The model under review builds one solid part; all positions refer to its coordinate system, in mm. A direction names the side the tool comes from. Coordinates: 2 decimals unless noted, no trailing zeros. Loops run counter-clockwise (first coordinate to the right, second up) from the corner with the lowest first, then second, coordinate; pieces in that order, holes last. Notation, with made-up numbers: (17, 11.5) -> (43, 11.5) arc R14 ccw to (43, 22.5) -> close; hole circle Ø5 at (23, 24.5). An arc over 180 degrees is marked (long way). One line per question, with ' | ' between items. Start each with the question number.
Autodesk Inventor part; units mm, degrees
ref_plane "XZ Plane" through (0, 0, 0) normal (0, 1, 0) x (-1, 0, 0)
ref_plane "XY Plane" through (0, 0, 0) normal (0, 0, 1) x (1, 0, 0)
sketch "Skizze1" plane through (0, 0, 0) normal (0, 0, 1) x (1, 0, 0)
  line L0 (-4.75, 4.75) -> (4.75, 4.75)
  line L1 (4.75, 4.75) -> (4.75, -4.75)
  line L2 (4.75, -4.75) -> (-4.75, -4.75)
  line L3 (-4.75, -4.75) -> (-4.75, 4.75)
  line L4 (-4.75, 4.75) -> (4.75, -4.75) construction
  line L5 (4.75, 4.75) -> (-4.75, -4.75) construction
  point P0 (0, 0)
  dimension "d0" = 9.5
  dimension "d1" = 9.5
extrude "Extrusion1" add sketch "Skizze1" along normal blind 3
sketch "Skizze2" plane through (0, 0, 3) normal (0, 0, 1) x (1, 0, 0)
  circle A0 centre (0, 0) radius 7.4
  dimension "d4" = 14.8
extrude "Extrusion2" add sketch "Skizze2" along normal blind 10
sketch "Skizze5" plane through (0, 0, 0) normal (0, 0, -1) x (-1, 0, 0)
  circle A0 centre (0, 0) radius 2
  dimension "d13" = 4
extrude "Extrusion5" cut sketch "Skizze5" against normal blind 5
sketch "Skizze6" plane through (0, 0, 13) normal (0, 0, 1) x (1, 0, 0)
  circle A0 centre (0, 0) radius 8.5
  dimension "d16" = 17
extrude "Extrusion6" add sketch "Skizze6" along normal blind 5
sketch "Skizze7" plane through (0, 0, 18) normal (0, 0, 1) x (1, 0, 0)
  circle A0 centre (0, 0) radius 4.9
  dimension "d19" = 9.8
extrude "Extrusion7" add sketch "Skizze7" along normal blind 36
sketch "Skizze8" plane through (0, 0, 54) normal (0, 0, 1) x (1, 0, 0)
  circle A0 centre (0, 0) radius 2
  dimension "d22" = 4
extrude "Extrusion8" cut sketch "Skizze8" against normal blind 5
properties part number "_3D-Druck"
1) Wall thickness on L1, parallel to Y at x = 0, z = 1.8; L2, parallel to Y at x = 0, z = 52.2; L3, parallel to Z at x = 6.5, y = -0.75: over which ranges is each line inside the solid? List them lowest first.
2) Consider section A-A, the plane x = 0. Write out the cut boundary in (y, z), plus the area to 3 significant figures.
3) Consider section C-C, the plane z = 49.5. Write out the cut boundary in (x, y).
4) Machinability: for faces 5 (the face through (4.75, 0, 1)), 6 (the face through (0, 4.75, 1)), 7 (the face through (-4.75, 0, 1)), 8 (the face through (0, -2, 2)), 9 (the face through (-1.062, 4.783, 35.748)), which of the approach directions +Z, -Z, +X, -X, +Y, -Y give a long, thin tool a straight path to every point of the face, cutting with its end or side? Answer none if there is none.
5) Consider section D-D, the plane z = 24.5. Write out the cut boundary in (x, y), plus the area to 3 significant figures.
6) Insertion check: pin 1 Ø2 at (x, y) = (3.5, -1) entering from -Z; pin 2 Ø3.5 at (y, z) = (-1.5, 1.5) entering from -X; pin 3 Ø2.5 at (x, y) = (0, 0) entering from +Z; pin 4 Ø1.5 at (y, z) = (-0.5, 19.5) entering from +X. Each pin has a flat end and moves straight along its axis. Give the tip position at first contact, or say it passes through.
7) Mouldability with a two-part tool opening along X and no side actions: class faces 1 (the face through (-1.604, 7.224, 7.93)), 2 (the face through (0, -2, 52)), 3 (the face through (0, 0, 49)), 4 (the face through (-2.2, 0.1, 0)) as +X half, -X half, draft (parallel to the pull), parting line (faces both ways), or undercut.
Filled sheet:
1) L1: -4.75 to -2, 2 to 4.75 | L2: -4.9 to -2, 2 to 4.9 | L3: 3 to 18
2) outline: (-8.5, 13) -> (-7.4, 13) -> (-7.4, 3) -> (-4.75, 3) -> (-4.75, 0) -> (-2, 0) -> (-2, 5) -> (2, 5) -> (2, 0) -> (4.75, 0) -> (4.75, 3) -> (7.4, 3) -> (7.4, 13) -> (8.5, 13) -> (8.5, 18) -> (4.9, 18) -> (4.9, 54) -> (2, 54) -> (2, 49) -> (-2, 49) -> (-2, 54) -> (-4.9, 54) -> (-4.9, 18) -> (-8.5, 18) -> close | area: 574 mm^2
3) outline: circle Ø9.8 at (0, 0); hole circle Ø4 at (0, 0)
4) face 5: -Z, +X, +Y, -Y | face 6: -Z, +X, -X, +Y | face 7: -Z, -X, +Y, -Y | face 8: -Z | face 9: +Z
5) outline: circle Ø9.8 at (0, 0) | area: 75.4 mm^2
6) pin 1: z = 0 | pin 2: x = -7.38 | pin 3: z = 49 | pin 4: x = 4.9
7) face 1: parting line | face 2: undercut | face 3: undercut | face 4: draft
